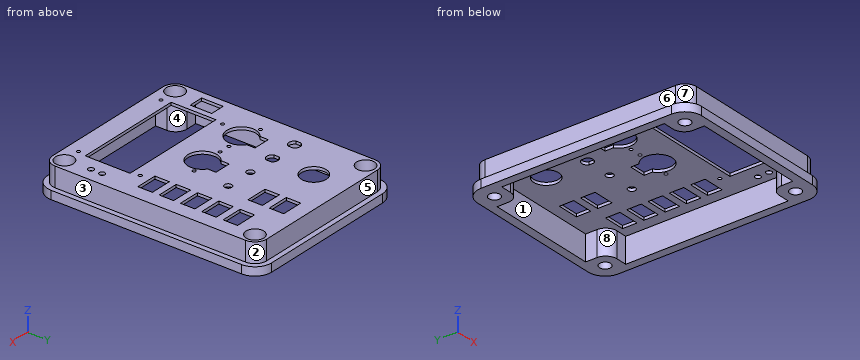
from build123d import *

# Parameters (mm, degrees)
SKETCH_W        = 155
SKETCH_H        = 200
PAD_DEPTH       = 25
POCKET_DEPTH    = 22.5
FILLET_R        = 15
SKETCH002_R     = 5
POCKET001_DEPTH = 25.001
SKETCH003_R     = 8
POCKET002_DEPTH = 16
POCKET003_DEPTH = 17.5
POCKET004_DEPTH = 17.5
SKETCH006_R     = 1.5
SKETCH006_W     = 97
SKETCH006_H     = 40
POCKET005_DEPTH = 2.501
SKETCH007_R     = 11.125
SKETCH007_R_2   = 1.5
SKETCH007_R_3   = 3.25
SKETCH007_R_4   = 2.5
SKETCH007_W     = 19.2
SKETCH007_H     = 12.9
SKETCH007_W_2   = 12.9
SKETCH007_H_2   = 19.2
POCKET006_DEPTH = 5


with BuildPart() as part:
    # Sketch → Pad (new body)
    with BuildSketch(Plane.XY):
        with Locations((77.5, 100)):
            Rectangle(SKETCH_W, SKETCH_H)
    extrude(amount=PAD_DEPTH)

    # Sketch001 (on Face5 of Pad) → Pocket (cut)
    with BuildSketch(Plane(origin=(0, 0, 0), x_dir=(1, 0, 0), z_dir=(0, 0, -1))):
        with BuildLine():
            ThreePointArc((17.500001, -27.5), (24.571081, -24.571055), (27.5, -17.499964))
            Line((27.5, -17.499964), (27.5, -7.5))
            Line((27.5, -7.5), (127.5, -7.5))
            Line((127.5, -7.5), (127.5, -17.500001))
            ThreePointArc((127.5, -17.500001), (130.428932, -24.571068), (137.499999, -27.5))
            Line((137.499999, -27.5), (147.5, -27.5))
            Line((147.5, -27.5), (147.5, -172.5))
            Line((147.5, -172.5), (137.499999, -172.5))
            ThreePointArc((137.499999, -172.5), (130.428932, -175.428932), (127.5, -182.499998))
            Line((127.5, -192.5), (127.5, -182.499998))
            Line((27.5, -192.5), (127.5, -192.5))
            Line((27.5, -182.499999), (27.5, -192.5))
            ThreePointArc((27.5, -182.499999), (24.571068, -175.428932), (17.500001, -172.5))
            Line((17.500001, -172.5), (7.5, -172.5))
            Line((7.5, -172.5), (7.5, -27.5))
            Line((7.5, -27.5), (17.500001, -27.5))
        make_face()
    extrude(amount=-POCKET_DEPTH, mode=Mode.SUBTRACT)

    # Fillet
    fillet_edges = [part.edges().sort_by_distance(p)[0] for p in [
        (155, 0, 12.5),
        (155, 200, 12.5),
        (0, 0, 12.5),
        (0, 200, 12.5),
    ]]
    fillet(fillet_edges, radius=FILLET_R)

    # Sketch002 (on Face2 of Fillet) → Pocket001 (cut, through all)
    with BuildSketch(Plane(origin=(0, 0, 0), x_dir=(1, 0, 0), z_dir=(0, 0, -1))):
        with Locations((15, -15)):
            Circle(SKETCH002_R)
        with Locations((140, -15)):
            Circle(SKETCH002_R)
        with Locations((140, -185)):
            Circle(SKETCH002_R)
        with Locations((15, -185)):
            Circle(SKETCH002_R)
    extrude(amount=-POCKET001_DEPTH, mode=Mode.SUBTRACT)

    # Sketch003 (on Face5 of Pocket001) → Pocket002 (cut)
    with BuildSketch(Plane.XY.offset(25)):
        with Locations((15, 185)):
            Circle(SKETCH003_R)
        with Locations((140, 185)):
            Circle(SKETCH003_R)
        with Locations((140, 15)):
            Circle(SKETCH003_R)
        with Locations((15, 15)):
            Circle(SKETCH003_R)
    extrude(amount=-POCKET002_DEPTH, mode=Mode.SUBTRACT)

    # Sketch004 (on Face5 of Pocket002) → Pocket003 (cut)
    with BuildSketch(Plane.XY.offset(25)):
        with BuildLine():
            ThreePointArc((15, 200), (4.393398, 195.606602), (0, 185))
            Line((0, 15), (0, 185))
            ThreePointArc((0, 15), (4.393398, 4.393398), (15, 0))
            Line((140, 0), (15, 0))
            ThreePointArc((140, 0), (150.606602, 4.393398), (155, 15))
            Line((155, 185), (155, 15))
            ThreePointArc((155, 185), (150.606602, 195.606602), (140, 200))
            Line((15, 200), (140, 200))
        make_face()
        with BuildLine():
            ThreePointArc((15, 195.5), (7.575379, 192.424621), (4.5, 185))
            Line((4.5, 185), (4.5, 15))
            ThreePointArc((4.5, 15), (7.575379, 7.575379), (15, 4.5))
            Line((15, 4.5), (140, 4.5))
            ThreePointArc((140, 4.5), (147.424621, 7.575379), (150.5, 15))
            Line((150.5, 15), (150.5, 184.999955))
            ThreePointArc((150.5, 184.999955), (147.424637, 192.424605), (140, 195.5))
            Line((15, 195.5), (140, 195.5))
        make_face(mode=Mode.SUBTRACT)
    extrude(amount=POCKET003_DEPTH, mode=Mode.SUBTRACT)

    # Sketch004 (on Face5 of Pocket002) → Pocket004 (cut)
    with BuildSketch(Plane.XY.offset(25)):
        with BuildLine():
            ThreePointArc((15, 200), (4.393398, 195.606602), (0, 185))
            Line((0, 15), (0, 185))
            ThreePointArc((0, 15), (4.393398, 4.393398), (15, 0))
            Line((140, 0), (15, 0))
            ThreePointArc((140, 0), (150.606602, 4.393398), (155, 15))
            Line((155, 185), (155, 15))
            ThreePointArc((155, 185), (150.606602, 195.606602), (140, 200))
            Line((15, 200), (140, 200))
        make_face()
        with BuildLine():
            ThreePointArc((15, 195.5), (7.575379, 192.424621), (4.5, 185))
            Line((4.5, 185), (4.5, 15))
            ThreePointArc((4.5, 15), (7.575379, 7.575379), (15, 4.5))
            Line((15, 4.5), (140, 4.5))
            ThreePointArc((140, 4.5), (147.424621, 7.575379), (150.5, 15))
            Line((150.5, 15), (150.5, 184.999955))
            ThreePointArc((150.5, 184.999955), (147.424637, 192.424605), (140, 195.5))
            Line((15, 195.5), (140, 195.5))
        make_face(mode=Mode.SUBTRACT)
    extrude(amount=-POCKET004_DEPTH, mode=Mode.SUBTRACT)

    # Sketch006 (on Face40 of Pocket004) → Pocket005 (cut, through all)
    with BuildSketch(Plane(origin=(0, 0, 22.5), x_dir=(1, 0, 0), z_dir=(0, 0, -1))):
        with Locations((31, -15)):
            Circle(SKETCH006_R)
        with Locations((124, -15)):
            Circle(SKETCH006_R)
        with Locations((124, -70)):
            Circle(SKETCH006_R)
        with Locations((31, -70)):
            Circle(SKETCH006_R)
        with Locations((77.5, -42.5)):
            Rectangle(SKETCH006_W, SKETCH006_H)
    extrude(amount=-POCKET005_DEPTH, mode=Mode.SUBTRACT)

    # Sketch007 (on Face40 of Pocket005) → Pocket006 (cut)
    with BuildSketch(Plane(origin=(0, 0, 22.5), x_dir=(1, 0, 0), z_dir=(0, 0, -1))):
        with Locations((47.5, -164.5)):
            Circle(SKETCH007_R)
        with Locations((20.5, -95.6)):
            Circle(SKETCH007_R_2)
        with Locations((95.5, -95.6)):
            Circle(SKETCH007_R_2)
        with Locations((53, -93.05)):
            Circle(SKETCH007_R_2)
        with Locations((63, -93.05)):
            Circle(SKETCH007_R_2)
        with Locations((72.5, -127.6)):
            Circle(SKETCH007_R_3)
        with Locations((97.5, -127.6)):
            Circle(SKETCH007_R_3)
        with Locations((138.5, -37.5)):
            Circle(SKETCH007_R_4)
        with Locations((138.5, -47.5)):
            Circle(SKETCH007_R_4)
        with Locations((127.9, -85.05)):
            Rectangle(SKETCH007_W, SKETCH007_H)
        with Locations((127.9, -123.05)):
            Rectangle(SKETCH007_W, SKETCH007_H)
        with Locations((127.9, -142.05)):
            Rectangle(SKETCH007_W, SKETCH007_H)
        with Locations((127.9, -161.05)):
            Rectangle(SKETCH007_W, SKETCH007_H)
        with Locations((127.9, -104.05)):
            Rectangle(SKETCH007_W, SKETCH007_H)
        with BuildLine():
            ThreePointArc((87.5, -101.41838), (80, -77.8), (72.5, -101.41838))
            Line((72.5, -101.41838), (72.5, -108.8))
            Line((72.5, -108.8), (87.5, -108.8))
            Line((87.5, -108.8), (87.5, -101.41838))
        make_face()
        with BuildLine():
            ThreePointArc((43.5, -101.41838), (36, -77.8), (28.5, -101.41838))
            Line((28.5, -101.41838), (28.5, -108.8))
            Line((28.5, -108.8), (43.5, -108.8))
            Line((43.5, -101.41838), (43.5, -108.8))
        make_face()
        with Locations((94.7, -157.05)):
            Rectangle(SKETCH007_W, SKETCH007_H)
        with Locations((94.7, -176.05)):
            Rectangle(SKETCH007_W, SKETCH007_H)
        with Locations((17.45, -45.1)):
            Rectangle(SKETCH007_W_2, SKETCH007_H_2)
        with BuildLine():
            Line((27, -125.420551), (27, -129.779449))
            ThreePointArc((18, -129.779449), (22.5, -132.6), (27, -129.779449))
            Line((18, -129.779449), (18, -125.420551))
            ThreePointArc((27, -125.420551), (22.5, -122.6), (18, -125.420551))
        make_face()
        with BuildLine():
            Line((52, -125.420551), (52, -129.779449))
            ThreePointArc((43, -129.779449), (47.5, -132.6), (52, -129.779449))
            Line((43, -129.779449), (43, -125.420551))
            ThreePointArc((52, -125.420551), (47.5, -122.6), (43, -125.420551))
        make_face()
    extrude(amount=-POCKET006_DEPTH, mode=Mode.SUBTRACT)


with BuildPart() as part_1:
    # Body placement: moved
    add(part.part.moved(Location((-15, -15, -25))))


solid = part_1.part
Build history of the part. All positions in model axes, mm. Face numbers are marked on the shaded views. A direction names the side the tool comes from. Coordinates: 2 decimals unless noted, no trailing zeros. Order: outer loops, then holes, each group sorted by start corner. A loop starts at its lowest first (then second) coordinate and runs counter-clockwise, first axis right, second up. Notation, with made-up numbers: (-15.5, 30.25) - (10.5, 30.25) arc R8 cw to (10.5, 35.25) - close; hole circle Ø4 at (-0.75, -39.5). An arc over 180 degrees is marked (long way). Put each result on its own line as item: value.
1. Drop flat-ended pins along their axis: P1, Ø3, axis at x = 83, z = -1.5, coming from the -Y side; P2, Ø2, axis at y = 130, z = -1, coming from the -X side; P3, Ø0.8, axis at x = 83, z = -1.5, coming from the +Y side; P4, Ø2, axis at x = 6, y = 41, coming from the +Z side. Give the stop position or say it passes through.
Answer sheet:
P1: stops at y = -10.5
P2: stops at x = -10.5
P3: stops at y = 180.5
P4: stops at z = 0
2. Pull direction Y, two halves, no side cores. Call the marked faces 1, 2, 3 and 4: pulls with the +Y half, pulls with the -Y half, needs draft (parallel to the pull), parting line crosses it, or undercut.
Answer sheet:
face 1: undercut
face 2: pulls with the +Y half
face 3: needs draft
face 4: undercut
3. Tool access for the marked faces 5, 6, 7 and 8: list every direction of +Z, -Z, +X, -X, +Y, -Y with a clear straight run to the whole face (end or side of a thin tool).
Answer sheet:
face 5: +Z, +X, -X, +Y
face 6: +Z, -X, +Y, -Y
face 7: +Z, -X, -Y
face 8: -Z
4. Saw through at C-C (y = 43). Write the cut outline in (x, z).
Answer sheet:
outline: (-15, -25) - (-7.5, -25) - (-7.5, -2.5) - (14, -2.5) - (14, 0) - (-10.5, 0) - (-10.5, -17.5) - (-15, -17.5) - close; (111, -2.5) - (132.5, -2.5) - (132.5, -25) - (140, -25) - (140, -17.5) - (135.5, -17.5) - (135.5, 0) - (111, 0) - close
5. Saw through at A-A (x = 65). Write the cut outline in (y, z), and give its area (4 significant figures).
Answer sheet:
outline: (-15, -25) - (-7.5, -25) - (-7.5, -2.5) - (7.5, -2.5) - (7.5, 0) - (-10.5, 0) - (-10.5, -17.5) - (-15, -17.5) - close; (47.5, -2.5) - (62.8, -2.5) - (62.8, 0) - (47.5, 0) - close; (93.8, -2.5) - (177.5, -2.5) - (177.5, -25) - (185, -25) - (185, -17.5) - (180.5, -17.5) - (180.5, 0) - (93.8, 0) - close
area: 502.5 mm^2
6. Saw through at B-B (z = -21.75). Write the cut outline in (x, y), and give its area (3 significant figures).
Answer sheet:
outline: (-15, 0) arc R15 ccw to (0, -15) - (125, -15) arc R15 ccw to (140, 0) - (140, 170) arc R15 ccw to (125, 185) - (0, 185) arc R15 ccw to (-15, 170) - close; hole (-7.5, 12.5) - (2.5, 12.5) arc R10 cw to (12.5, 2.5) - (12.5, -7.5) - (112.5, -7.5) - (112.5, 2.5) arc R10 cw to (122.5, 12.5) - (132.5, 12.5) - (132.5, 157.5) - (122.5, 157.5) arc R10 cw to (112.5, 167.5) - (112.5, 177.5) - (12.5, 177.5) - (12.5, 167.5) arc R10 cw to (2.5, 157.5) - (-7.5, 157.5) - close; hole circle Ø10 at (0, 0); hole circle Ø10 at (0, 170); hole circle Ø10 at (125, 0); hole circle Ø10 at (125, 170)
area: 6,110 mm^2
7. Probe line 1 along X through (y, z) = (75.8, -1.35); line 2 along Y through (x, z) = (0, -7.5); line 3 along X through (y, z) = (104, -4.5). List the from-to ranges inside material, lowest first. Write a range as [from, to].
Answer sheet:
line 1: x = [-10.5, 8], [34, 52], [78, 103.3], [122.5, 135.5]
line 2: y = [-10.5, -8], [8, 12.5], [157.5, 162], [178, 180.5]
line 3: x = [-10.5, -7.5], [132.5, 135.5]
